from build123d import *

# Parameters (mm, degrees)
F0_R     = 5.5
F1_DEPTH = 5


with BuildPart() as f1:
    # F0 (on Top) → F1 (new body)
    with BuildSketch(Plane.XY):
        with BuildLine():
            Line((-17.840159, 19.089536), (-6.065941, 5.21578))
            ThreePointArc((-6.065941, 5.21578), (0, -8), (6.065941, 5.21578))
            Line((6.065941, 5.21578), (17.840159, 19.089536))
            ThreePointArc((17.840159, 19.089536), (27.176471, 32.022483), (15.934059, 20.707183))
            Line((15.934059, 20.707183), (4.159841, 6.833427))
            ThreePointArc((4.159841, 6.833427), (0, 8), (-4.159841, 6.833427))
            Line((-4.159841, 6.833427), (-15.934059, 20.707183))
            ThreePointArc((-15.934059, 20.707183), (-27.176471, 32.022483), (-17.840159, 19.089536))
        make_face()
        Circle(F0_R, mode=Mode.SUBTRACT)
        with Locations((-22, 25.922963)):
            Circle(F0_R, mode=Mode.SUBTRACT)
        with Locations((22, 25.922963)):
            Circle(F0_R, mode=Mode.SUBTRACT)
    extrude(amount=F1_DEPTH)


solid = f1.part
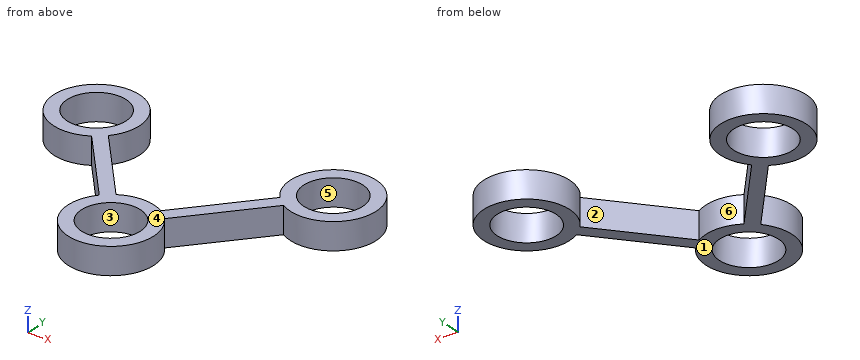
Model file for the job. Use its own axes, mm. Face numbers are marked on the shaded views. A direction names the side the tool comes from. Give positions to 0.01 mm unless a question says otherwise; leave off trailing zeros. Order: outer loops, then holes, each group sorted by start corner. A loop starts at its lowest first (then second) coordinate and runs counter-clockwise, first axis right, second up. Notation, with made-up numbers: M 50.25,25 L 59.25,25 A6 cw 59.25,33 Z; hole C -34,80.25 d6. An arc over 180 degrees is marked long. Put each result on its own line as item: value. Start each with the question number.
(1) Band-saw the part on C-C on z = 2.7. Give the cut face in (x, y), then the cut area to 3 significant figures.
(2) Drill centre lines: L1, parallel to Y at x = -22, z = 2.55; L2, parallel to X at y = 22.5, z = 0.4; L3, parallel to Y at x = 0, z = 3.4. Where is each one in solid material? Low to high. Write a range as [from, to].
(3) Tool access for the marked faces 1 and 2: list every direction of +Z, -Z, +X, -X, +Y, -Y with a clear straight run to the whole face (end or side of a thin tool).
(4) Band-saw the part on A-A on x = 0. Give the cut face in (y, z), then the cut area to 3 significant figures.
(5) Band-saw the part on D-D on x = 12. Give the cut face in (y, z).
(6) Pull direction Y, two halves, no side cores. Call the marked faces 3, 4, 5 and 6: released by +Y, released by -Y, zero draft, split by the parting line, or undercut.
(7) Pin check, flat tips, straight feed: pin 1 Ø2 at (x, y) = (-3, 3) entering from -Z; pin 2 Ø6 at (x, y) = (10, 8) entering from +Z; pin 3 Ø1.5 at (y, z) = (3.5, 1.5) entering from -X. Stop position of each tip, or through.
Results below:
1. outline: M -17.84,19.09 L -6.07,5.22 A8 ccw long 6.07,5.22 L 17.84,19.09 A8 ccw long 15.93,20.71 L 4.16,6.83 A8 ccw -4.16,6.83 L -15.93,20.71 A8 ccw long Z; hole C -22,25.92 d11; hole C 0,0 d11; hole C 22,25.92 d11
1. area: 408 mm2
2. L1: y = [17.92, 20.42], [31.42, 33.92]
2. L2: x = [-29.23, -26.31], [-17.69, -14.77], [14.77, 17.69], [26.31, 29.23]
2. L3: y = [-8, -5.5], [5.5, 8]
3. face 1: -Z, +X, -X, +Y, -Y
3. face 2: +Z, -Z
4. outline: M -8,0 L -5.5,0 L -5.5,5 L -8,5 Z; M 5.5,0 L 8,0 L 8,5 L 5.5,5 Z
4. area: 25.0 mm2
5. outline: M 12.21,0 L 16.07,0 L 16.07,5 L 12.21,5 Z
6. face 3: undercut
6. face 4: zero draft
6. face 5: undercut
6. face 6: released by +Y
7. pin 1: passes through
7. pin 2: stops at z = 5
7. pin 3: stops at x = -7.51
